The listing builds one solid part. Answer for the finished solid, in the listing's coordinates (mm). A direction names the side the tool comes from. Round coordinates to 2 decimals unless told otherwise and drop trailing zeros. Loops run counter-clockwise (first coordinate to the right, second up) from the corner with the lowest first, then second, coordinate; pieces in that order, holes last. Notation, with made-up numbers: (54, 67) - (112, 67) arc R23 ccw to (112, 89) - close; hole circle Ø8 at (88, 69). An arc over 180 degrees is marked (long way). One line per item, written item: value.
```python
from build123d import *

# Parameters (mm, degrees)
F1_DEPTH    = 48
F2_DEPTH    = 10
F3_T1_DEPTH = 32.1050237641
F4_T1_DEPTH = 32.1050237641
F5_W        = 28
F5_H        = 5
F6_DEPTH    = 5
F5_R        = 6
F7_DEPTH    = 3
F8_DEPTH    = 25


# Not quite as in the source:
# - a fillet or chamfer that OpenCascade refuses, or shapes differently, is made with other operations: its cross-section is extruded or revolved along the edge and cut away or added


with BuildPart() as f1:
    # F0 (on Top) → F1 (new body)
    with BuildSketch(Plane.XY):
        Polygon((31, -8.1050237641), (31, 24), (21, 24), (21, 1.8949762359), (-21, 1.8949762359), (-21, 24), (-31, 24), (-31, -8.1050237641), align=None)
    extrude(amount=F1_DEPTH)

    # F0 (on Top) → F2 (join)
    with BuildSketch(Plane.XY):
        with BuildLine():
            Line((-40, -24), (40, -24))
            ThreePointArc((40, -24), (44.2426406871, -22.2426406871), (46, -18))
            Line((46, -18), (46, 24))
            Line((46, 24), (31, 24))
            Line((31, 24), (31, -8.1050237641))
            Line((31, -8.1050237641), (-31, -8.1050237641))
            Line((-31, -8.1050237641), (-31, 24))
            Line((-31, 24), (-46, 24))
            Line((-46, 24), (-46, -18))
            ThreePointArc((-46, -18), (-44.2426406871, -22.2426406871), (-40, -24))
        make_face()
        Polygon((31, -8.1050237641), (31, 24), (21, 24), (21, 1.8949762359), (-21, 1.8949762359), (-21, 24), (-31, 24), (-31, -8.1050237641), align=None)
    extrude(amount=F2_DEPTH)

    # F3: fillet of radius 25 on 1 edges, made by hand

    # F3_s2 → F3_t1 (join)
    with BuildSketch(Plane.XZ.offset(-24)):
        with BuildLine():
            ThreePointArc((46, 10), (35.0834993366, 19.2198145372), (31, 32.9128784748))
            Line((31, 32.9128784748), (31, 10))
            Line((31, 10), (46, 10))
        make_face()
    extrude(amount=F3_T1_DEPTH)

    # F4: fillet of radius 25 on 1 edges, made by hand

    # F4_s2 → F4_t1 (join)
    with BuildSketch(Plane.XZ.offset(-24)):
        with BuildLine():
            ThreePointArc((-31, 32.9128784748), (-35.0834993366, 19.2198145372), (-46, 10))
            Line((-46, 10), (-31, 10))
            Line((-31, 10), (-31, 32.9128784748))
        make_face()
    extrude(amount=F4_T1_DEPTH)

    # F5 (on face) → F6 (join)
    with BuildSketch(Plane.XZ.offset(8.1050237641)):
        with Locations((0, 12.5)):
            Rectangle(F5_W, F5_H)
    extrude(amount=F6_DEPTH)

    # F5 (on face) → F7 (join)
    with BuildSketch(Plane.XZ.offset(8.1050237641)):
        with BuildLine():
            Line((14, 15), (14, 29))
            ThreePointArc((14, 29), (0, 43), (-14, 29))
            Line((-14, 29), (-14, 15))
            Line((-14, 15), (14, 15))
        make_face()
        with Locations((0, 29)):
            Circle(F5_R, mode=Mode.SUBTRACT)
    extrude(amount=F7_DEPTH)

    # F8 (cut): a face of the model
    f8_faces = [f1.faces().sort_by_distance(p)[0] for p in [
        (0, -8.1050237641, 29),
    ]]
    extrude(f8_faces, amount=-F8_DEPTH, mode=Mode.SUBTRACT)


solid = f1.part
```
1) A cutting plane is placed at A-A on x = 0. Give the vertices of the cut face in (y, z), and give its area (3 significant figures).
Final values:
outline: (-24, 0) - (1.89, 0) - (1.89, 23) - (-11.11, 23) - (-11.11, 15) - (-13.11, 15) - (-13.11, 10) - (-24, 10) - close; (-11.11, 35) - (1.89, 35) - (1.89, 48) - (-8.11, 48) - (-8.11, 43) - (-11.11, 43) - close
area: 592 mm2
2) A cutting plane is placed at C-C on z = 7. Give the vertices of the cut face in (x, y), and give its area (3 significant figures).
Final values:
outline: (-46, -18) arc R6 ccw to (-40, -24) - (40, -24) arc R6 ccw to (46, -18) - (46, 24) - (21, 24) - (21, 1.89) - (-21, 1.89) - (-21, 24) - (-46, 24) - close
area: 3,470 mm2
3) For a pull along X with two mould halves and no side action, classify faces 1 (the flat face through (-21, 13, 24)), 2 (the cylindrical face through (44.196, -22.289, 4.93)), 3 (the flat face through (31, 24, 19)) as released by +X, released by -X, zero draft, split by the parting line, or undercut.
Final values:
face 1: undercut
face 2: released by +X
face 3: zero draft
4) Consider L1, parallel to Z at x = 0, y = -10; L2, parallel to Z at x = 0, y = -1; L3, parallel to X at y = 6, z = 9. Determine where each line is inside the solid, lowest interval first.
Final values:
L1: 0 to 23, 35 to 43
L2: 0 to 23, 35 to 48
L3: -46 to -21, 21 to 46
5) For faces 4 (the flat face through (31, 8, 40)), 5 (the flat face through (21, 13, 24)), 6 (the flat face through (0, -13.105, 13)), determine the directions among +Z, -Z, +X, -X, +Y, -Y from which every point of the face is accessible in a straight line to the end or side of a thin tool.
Final values:
face 4: +Z, +X, +Y, -Y
face 5: +Z, -Z, +Y
face 6: +Z, +X, -X, -Y
6) A cutting plane is placed at B-B on y = 18.5. Give the vertices of the cut face in (x, z), and give its area (3 significant figures).
Final values:
outline: (-46, 0) - (-21, 0) - (-21, 48) - (-31, 48) - (-31, 32.91) arc R25 cw to (-46, 10) - close; (21, 0) - (46, 0) - (46, 10) arc R25 cw to (31, 32.91) - (31, 48) - (21, 48) - close
area: 1,450 mm2
7) Each of these flat-tipped pins is pushed along its axis until it touches: pin 1 Ø3 at (y, z) = (2, 33.5) entering from -X; pin 2 Ø4 at (x, y) = (26, 5) entering from -Z; pin 3 Ø12 at (y, z) = (-4, 23) entering from -X; pin 4 Ø6 at (x, z) = (-27.5, 38) entering from -Y (3 decimals). Where does it stop, or does it pass through?
Final values:
pin 1: x = -31.02
pin 2: z = 0
pin 3: x = -36.72
pin 4: y = -8.105
8) A cutting plane is placed at D-D on z = 24.5. Give the vertices of the cut face in (x, y), and give its area (3 significant figures).
Final values:
outline: (-32.46, -8.11) - (-14, -8.11) - (-14, -11.11) - (-3.97, -11.11) - (-3.97, 1.89) - (-21, 1.89) - (-21, 24) - (-32.46, 24) - close; (3.97, -11.11) - (14, -11.11) - (14, -8.11) - (32.46, -8.11) - (32.46, 24) - (21, 24) - (21, 1.89) - (3.97, 1.89) - close
area: 1,140 mm2
